Print and shaded views of the part. All mm, measured from the part's lowest x, y and z. Round coordinates to 2 decimals unless told otherwise and drop trailing zeros. Write each loop counter-clockwise with the first axis right and the second up, starting at its lowest first coordinate (ties: lowest second). Pieces come first, ordered by that corner, then holes. Notation, with made-up numbers: (32, 50.25) -> (88, 50.25) arc R15 ccw to (88, 79.25) -> close; hole circle Ø1 at (-4, 69). An arc over 180 degrees is marked (long way). Use CSV: the item, a comma, the result in double quotes. Start each with the question number.
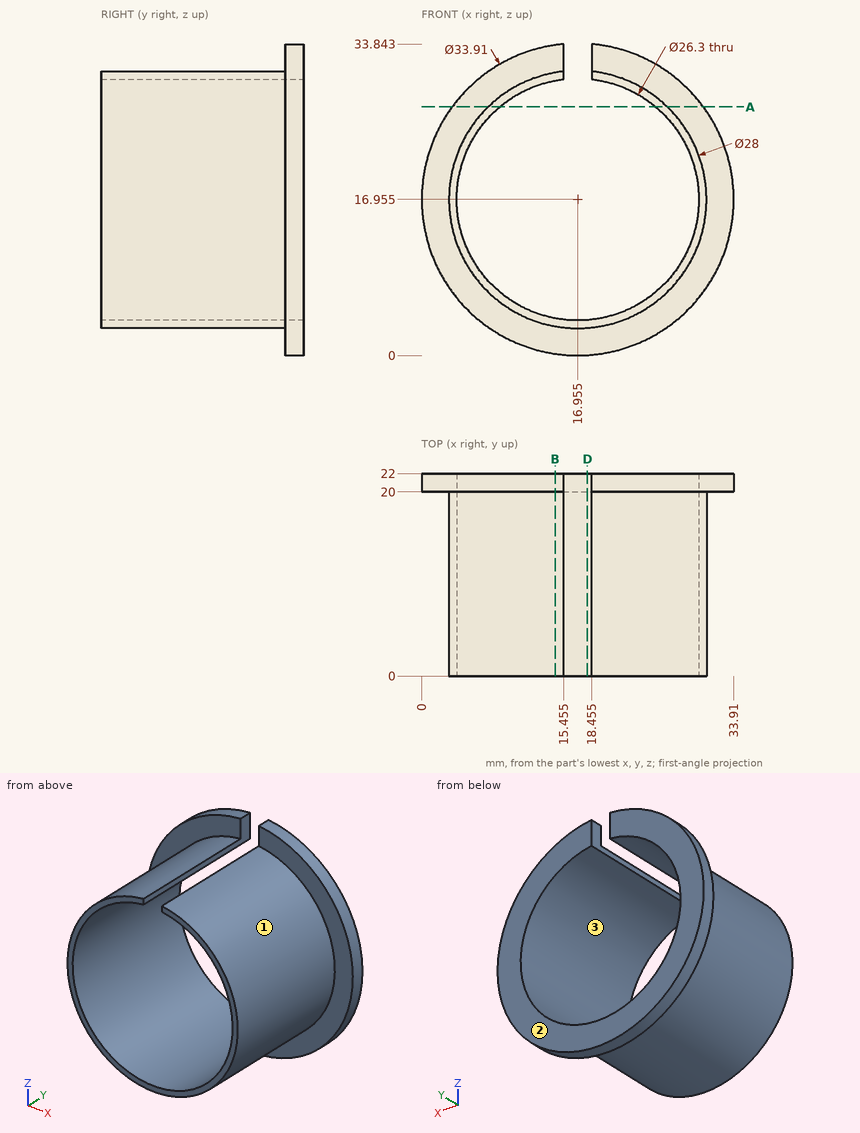
1. Band-saw the part on D-D (x = 18). List the corners of the cut face in (y, z).
2. Band-saw the part on B-B (x = 14.5). List the corners of the cut face in (y, z).
3. Pull direction Z, two halves, no side cores. Call the marked faces 1, 2 and 3: released by +Z, released by -Z, zero draft, split by the parting line, or undercut.
4. Flat gauge pins, fed straight in: pin 1 (2 mm diameter, centred on y = 13.5, z = 11.5, fed in from -X); pin 2 (4 mm diameter, centred on y = 15, z = 31, fed in from +X); pin 3 (1 mm diameter, centred on x = 25, y = 10, fed in from -Z); pin 4 (3 mm diameter, centred on x = 15, z = 28.5, fed in from +Y). Where does each tip first touch, or does it go through?
5. Band-saw the part on A-A (z = 27). List the corners of the cut face in (x, y).
6. Drill centre lines: line 1 along X through (y, z) = (6, 9.5) (1 decimal); line 2 along Y through (x, z) = (8.5, 5.5); line 3 along X through (y, z) = (2.75, 24.5) (1 decimal). Where is each one in solid material? Low to high. Write a range as [from, to].
Answers below:
1,outline,"(0, 2.99) -> (20, 2.99) -> (20, 0.03) -> (22, 0.03) -> (22, 3.85) -> (0, 3.85) -> close"
2,outline,"(0, 3.17) -> (20, 3.17) -> (20, 0.18) -> (22, 0.18) -> (22, 4.04) -> (0, 4.04) -> close; (0, 29.87) -> (22, 29.87) -> (22, 33.73) -> (20, 33.73) -> (20, 30.74) -> (0, 30.74) -> close"
3,face 1,"split by the parting line"
3,face 2,"zero draft"
3,face 3,"undercut"
4,pin 1,"stops at x = 3.68"
4,pin 2,"stops at x = 24.09"
4,pin 3,"stops at z = 5.16"
4,pin 4,"stops at y = 22"
5,outline,"(3.3, 20) -> (7.2, 20) -> (7.2, 0) -> (8.47, 0) -> (8.47, 22) -> (3.3, 22) -> close; (25.44, 0) -> (26.71, 0) -> (26.71, 20) -> (30.61, 20) -> (30.61, 22) -> (25.44, 22) -> close"
6,line 1,"x = [5.1, 6.1], [27.8, 28.8]"
6,line 2,"y = [20, 22]"
6,line 3,"x = [5.2, 6.2], [27.7, 28.7]"
